For this review, use the dimensioned drawing (mm, ordinates from the lowest corner) and the shaded views. Coordinates: 2 decimals unless noted, no trailing zeros. Loops run counter-clockwise (first coordinate to the right, second up) from the corner with the lowest first, then second, coordinate; pieces in that order, holes last. Notation, with made-up numbers: (81, -26.5) -> (94, -26.5) arc R26 ccw to (94, -6.5) -> close; hole circle Ø2 at (79.5, 53). An arc over 180 degrees is marked (long way). Answer as a JSON object with one key per item and string values.
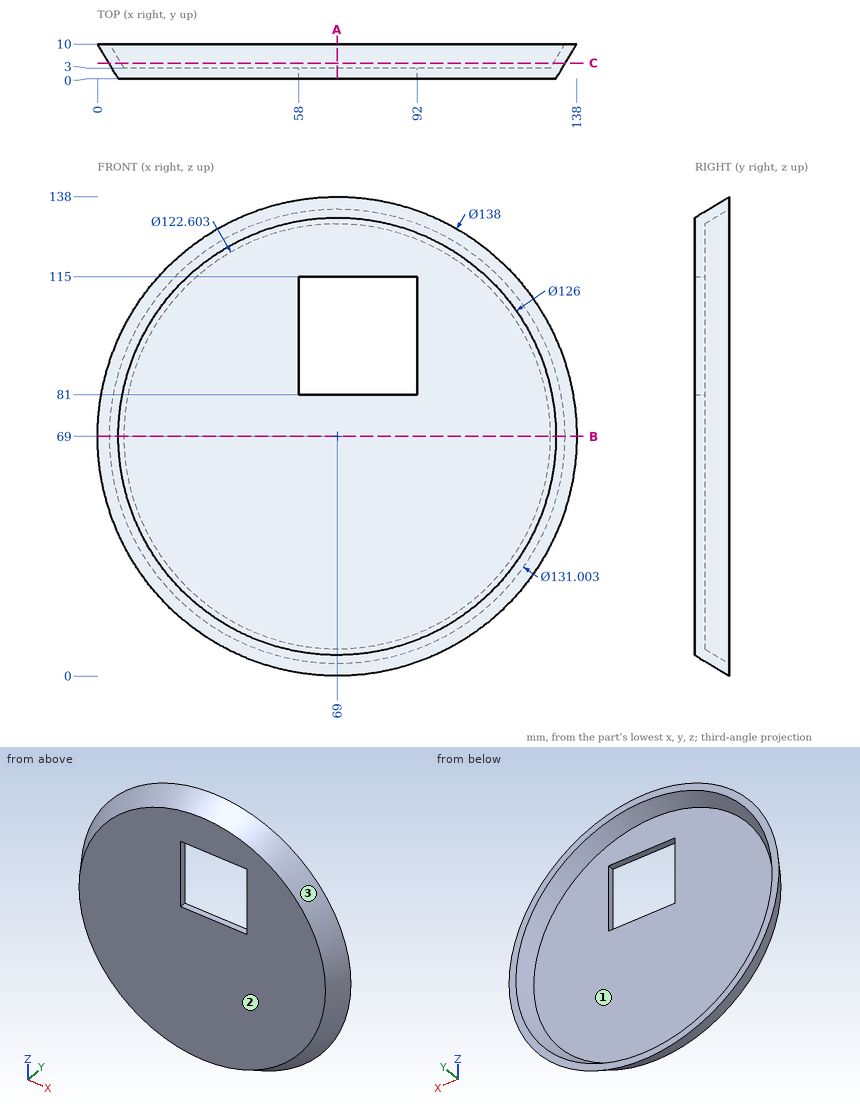
1) Add section A-A, the plane x = 69. Give the boundary of the cut face in (y, z).
Completed:
{"outline": "(0, 6) -> (10, 0) -> (10, 3.5) -> (3, 7.7) -> (3, 81) -> (0, 81) -> close; (0, 115) -> (3, 115) -> (3, 130.3) -> (10, 134.5) -> (10, 138) -> (0, 132) -> close"}
2) Add section B-B, the plane z = 69. Give the boundary of the cut face in (x, y).
Completed:
{"outline": "(0, 10) -> (6, 0) -> (132, 0) -> (138, 10) -> (134.5, 10) -> (130.3, 3) -> (7.7, 3) -> (3.5, 10) -> close"}
3) Wall thickness on probe 1 along X at (y, z) = (8.75, 98.5) (1 decimal); probe 2 along X at (y, z) = (4.75, 29); probe 3 along Y at (x, z) = (51, 113): over which ranges is each line inside the solid? List them lowest first.
Completed:
{"probe 1": "7.5 to 11.4, 126.6 to 130.5", "probe 2": "16.69 to 21.17, 116.83 to 121.31", "probe 3": "0 to 3"}
4) Add section C-C, the plane y = 4.5. Give the boundary of the cut face in (x, z).
Completed:
{"outline": "circle Ø131.4 at (69, 69); hole circle Ø124.4 at (69, 69)"}
5) Clearance check with flat-ended pins moving along their axes: pin 1 Ø10 at (x, z) = (56.5, 57.5) entering from -Y; pin 2 Ø1.5 at (y, z) = (5.5, 59) entering from -X; pin 3 Ø1.5 at (x, z) = (53, 71) entering from +Y; pin 4 Ø0.9 at (y, z) = (1, 94.5) entering from +X. State where each tip first meets the part, or that it passes through.
Completed:
{"pin 1": "y = 0", "pin 2": "x = 2.99", "pin 3": "y = 3", "pin 4": "x = 127.62"}
6) The part is to be moulded in two halves that separate along Z. For the marked faces 1, 2 and 3, say which applies: pulls with the +Z half, pulls with the -Z half, needs draft (parallel to the pull), parting line crosses it, or undercut.
Completed:
{"face 1": "undercut", "face 2": "needs draft", "face 3": "parting line crosses it"}
